For this review, take the finished solid that the model builds, in its own axes (mm). A direction names the side the tool comes from. Coordinates: 2 decimals unless noted, no trailing zeros. Write each loop counter-clockwise with the first axis right and the second up, starting at its lowest first coordinate (ties: lowest second). Pieces come first, ordered by that corner, then holes.
```python
from build123d import *

# Parameters (mm, degrees)
SALIENTE_EXTRUIR1_DEPTH = 3


with BuildPart() as part:
    # Croquis1 → Saliente-Extruir1 (new body)
    with BuildSketch(Plane.XY):
        with BuildLine():
            Line((0, 22.001027223), (-5, 22.001027223))
            Line((-5, 22.001027223), (-5, 12.001027223))
            ThreePointArc((-5, 12.001027223), (-4.121320344, 9.87970688), (-2, 9.001027223))
            Line((-2, 9.001027223), (7, 9.001027223))
            ThreePointArc((7, 9.001027223), (9.121320344, 9.87970688), (10, 12.001027223))
            Line((10, 12.001027223), (10, 19.001027223))
            Line((10, 19.001027223), (10, 22.001027223))
            Line((10, 22.001027223), (5, 22.001027223))
            Line((5, 22.001027223), (5, 19.001027223))
            Line((5, 19.001027223), (0, 19.001027223))
            Line((0, 19.001027223), (0, 22.001027223))
        make_face()
    extrude(amount=SALIENTE_EXTRUIR1_DEPTH)


solid = part.part
```
Q1. Tool access review of faces 1 (the flat face through (2, 16, 3)), 2 (the flat face through (5, 21, 1)): name each direction out of +Z, -Z, +X, -X, +Y, -Y from which nothing blocks a thin tool from reaching the whole face with its end or side.
Ans:
face 1: +Z, +X, -X, +Y, -Y
face 2: +Z, -Z, +Y
Q2. Add section A-A (z = 1.1). State the section outline as (x, y) points.
Ans:
outline: (-5, 12) arc R3 ccw to (-2, 9) - (7, 9) arc R3 ccw to (10, 12) - (10, 22) - (5, 22) - (5, 19) - (0, 19) - (0, 22) - (-5, 22) - close
Q3. Draft analysis for pull direction X (two halves, no side actions). For faces 3 (the flat face through (-2, 22.001, 1)), 4 (the flat face through (3, 19.001, 1)), 5 (the flat face through (10, 17, 1)), state which applies: +X half, -X half, draft (parallel to the pull), parting line (faces both ways), or undercut.
Ans:
face 3: draft
face 4: undercut
face 5: +X half
Q4. Add section B-B (x = 4). State the section outline as (y, z) points.
Ans:
outline: (9, 0) - (19, 0) - (19, 3) - (9, 3) - close
Q5. For probe 1 along Y at (x, z) = (3, 0.95); probe 2 along X at (y, z) = (19.5, 2.3); probe 3 along Y at (x, z) = (-4.25, 2.6), list the stretches that pass through material, from the lowest coordinate up.
Ans:
probe 1: y = 9 to 19
probe 2: x = -5 to 0, 5 to 10
probe 3: y = 10.02 to 22
Q6. Clearance check with flat-ended pins moving along their axes: pin 1 Ø1 at (x, y) = (2, 12.5) entering from -Z; pin 2 Ø0.9 at (x, z) = (3.5, 2) entering from +Y. State where each tip first meets the part, or that it passes through.
Ans:
pin 1: stops at z = 0
pin 2: stops at y = 19
